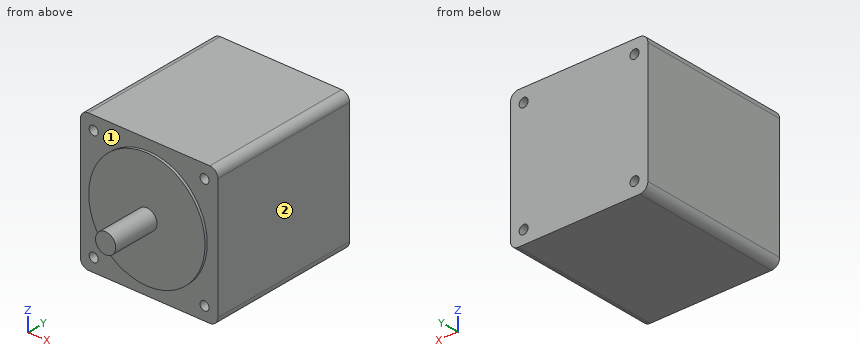
```python
from build123d import *

# Parameters (mm, degrees)
F0_R     = 2.8321
F1_DEPTH = 95.25
F2_R     = 36.5125
F3_DEPTH = 1.5875
F4_R     = 6.35
F5_DEPTH = 29.845


with BuildPart() as f1:
    # F0 (on Front) → F1 (new body)
    with BuildSketch(Plane.XZ):
        with BuildLine():
            ThreePointArc((0, 5.08), (1.487898, 1.487898), (5.08, 0))
            Line((5.08, 0), (81.28, 0))
            ThreePointArc((81.28, 0), (84.872102, 1.487898), (86.36, 5.08))
            Line((86.36, 5.08), (86.36, 81.28))
            ThreePointArc((86.36, 81.28), (84.872102, 84.872102), (81.28, 86.36))
            Line((81.28, 86.36), (5.08, 86.36))
            ThreePointArc((5.08, 86.36), (1.487898, 84.872102), (0, 81.28))
            Line((0, 81.28), (0, 5.08))
        make_face()
        with Locations((8.372527, 8.372527)):
            Circle(F0_R, mode=Mode.SUBTRACT)
        with Locations((77.987473, 8.372527)):
            Circle(F0_R, mode=Mode.SUBTRACT)
        with Locations((8.372527, 77.987473)):
            Circle(F0_R, mode=Mode.SUBTRACT)
        with Locations((77.987473, 77.987473)):
            Circle(F0_R, mode=Mode.SUBTRACT)
    extrude(amount=-F1_DEPTH)

    # F2 (on face) → F3 (join)
    with BuildSketch(Plane.XZ):
        with Locations((43.18, 43.18)):
            Circle(F2_R)
    extrude(amount=F3_DEPTH)

    # F4 (on face) → F5 (join)
    with BuildSketch(Plane.XZ.offset(1.5875)):
        with Locations((43.18, 43.18)):
            Circle(F4_R)
    extrude(amount=F5_DEPTH)


solid = f1.part
```
Geometry: final body of the model. Coordinates: model frame, mm. Face numbers are marked on the shaded views. A direction names the side the tool comes from. Coordinates: 2 decimals unless noted, no trailing zeros. Order: outer loops, then holes, each group sorted by start corner. A loop starts at its lowest first (then second) coordinate and runs counter-clockwise, first axis right, second up. Notation, with made-up numbers: (-11.75, 70) - (43.25, 70) arc R20 cw to (43.25, 108) - close; hole circle Ø7 at (7, 51). An arc over 180 degrees is marked (long way). Return JSON: item names as keys, results as strings. Group by question number.
1. Material intervals for line 1 along Z through (x, y) = (76.5, 45); line 2 along Z through (x, y) = (10.5, 17.5); line 3 along Y through (x, z) = (82, 21), sorted ascending. Write a range as [from, to].
2. Set-up query: the marked faces 1 and 2. Return all of +Z, -Z, +X, -X, +Y, -Y with unobstructed straight access to the full face (end or side cutting, diameter ignored); none if empty.
3. Cut plane B-B (x = 43.18). Output: boundary loops of the cut face in (y, z), plus the area to 3 significant figures.
4. Cut plane C-C (y = 53). Output: boundary loops of the cut face in (x, z).
5. Pin query (flat end, axial travel): pin 1 (3 mm diameter, centred on y = -10, z = 48, fed in from -X); pin 2 (5 mm diameter, centred on x = 52, z = 52, fed in from -Y); pin 3 (9 mm diameter, centred on x = 77.99, z = 77.99, fed in from -Y). Return the tip coordinate at first contact, or that it passes through.
6. Cut plane A-A (z = 43.18). Output: boundary loops of the cut face in (x, y).
7. Cut plane D-D (y = -3.5). Output: boundary loops of the cut face in (x, z).
Resolved:
{
 "1": {"line 1": "z = [0, 5.96], [10.78, 75.58], [80.4, 86.36]", "line 2": "z = [0, 6.5], [10.24, 76.12], [79.86, 86.36]", "line 3": "y = [0, 95.25]"},
 "2": {"face 1": "-Y", "face 2": "+Z, -Z, +X, +Y, -Y"},
 "3": {"outline": "(-31.43, 36.83) - (-1.59, 36.83) - (-1.59, 6.67) - (0, 6.67) - (0, 0) - (95.25, 0) - (95.25, 86.36) - (0, 86.36) - (0, 79.69) - (-1.59, 79.69) - (-1.59, 49.53) - (-31.43, 49.53) - close", "area": "8,720 mm²"},
 "4": {"outline": "(0, 5.08) arc R5.08 ccw to (5.08, 0) - (81.28, 0) arc R5.08 ccw to (86.36, 5.08) - (86.36, 81.28) arc R5.08 ccw to (81.28, 86.36) - (5.08, 86.36) arc R5.08 ccw to (0, 81.28) - close; hole circle Ø5.66 at (8.37, 8.37); hole circle Ø5.66 at (8.37, 77.99); hole circle Ø5.66 at (77.99, 8.37); hole circle Ø5.66 at (77.99, 77.99)"},
 "5": {"pin 1": "stops at x = 37.77", "pin 2": "stops at y = -1.59", "pin 3": "stops at y = 0"},
 "6": {"outline": "(0, 0) - (6.67, 0) - (6.67, -1.59) - (36.83, -1.59) - (36.83, -31.43) - (49.53, -31.43) - (49.53, -1.59) - (79.69, -1.59) - (79.69, 0) - (86.36, 0) - (86.36, 95.25) - (0, 95.25) - close"},
 "7": {"outline": "circle Ø12.7 at (43.18, 43.18)"}
}
